Build history of the part. All positions in model axes, mm. A direction names the side the tool comes from. Round coordinates to 2 decimals unless told otherwise and drop trailing zeros. Order: outer loops, then holes, each group sorted by start corner. A loop starts at its lowest first (then second) coordinate and runs counter-clockwise, first axis right, second up. Notation, with made-up numbers: M 32.5,39 L 63.5,39 A33 cw 63.5,69 Z; hole C 25,27.25 d8. An arc over 180 degrees is marked long. One line per item, written item: value. Start each with the question number.
Item 1: Band-saw the part on B-B, the plane z = 0. Give the number of separate pieces and of enclosed holes in the cut face, then the cut area to 3 significant figures.
Item 2: Tool access for faces 4 (the cylindrical face through (3, 30, 0)), 5 (the flat face through (10, 1, 7)): list every direction of +Z, -Z, +X, -X, +Y, -Y with a clear straight run to the whole face (end or side of a thin tool).
Item 3: Band-saw the part on C-C, the plane x = 7. Write the cut outline in (y, z), then the cut area to 3 significant figures.
Item 4: Band-saw the part on D-D, the plane y = 0. Write the cut outline in (x, z).
Item 5: Probe L1, parallel to Y at x = 7.8, z = 0; L2, parallel to Y at x = 2, z = -3.5; L3, parallel to Y at x = 2.4, z = -25. List the from-to ranges inside material, lowest first.
Item 6: Two-plate mould, pull along Y, no slides. Class faces 1 (the flat face through (5, -43, 0)), 2 (the flat face through (5, -1, 31)), 3 (the cylindrical face through (2.71, -4.88, -1.08)): +Y half, -Y half, draft (parallel to the pull), parting line (faces both ways), or undercut.
Item 7: Band-saw the part on A-A, the plane y = 25. Write the cut outline in (x, z), then the cut area to 3 significant figures.
Item 8: Pin check, flat tips, straight feed: pin 1 (5 mm diameter, centred on y = -19, z = 0, fed in from +X); pin 2 (6 mm diameter, centred on y = 0, z = 25, fed in from -X). Stop position of each tip, or through.
```python
from build123d import *

# Parameters (mm, degrees)
SKETCH_1_W                = 62
SKETCH_1_H                = 86
EXTRUDE_1_DEPTH           = 10
CHAMFER_1_SIZE            = 1
HOLE_WIZARD_1_D           = 5.5
HOLE_WIZARD_1_CBORE_D     = 10
HOLE_WIZARD_1_CBORE_DEPTH = 5.5
HOLE_WIZARD_M5_1_D        = 4.2


with BuildPart() as part:
    # 草图1 → 凸台-拉伸1 (new body)
    with BuildSketch(Plane(origin=(0, 0, 0), x_dir=(0, 0, -1), z_dir=(1, 0, 0))):
        Rectangle(SKETCH_1_W, SKETCH_1_H)
    extrude(amount=EXTRUDE_1_DEPTH)

    # 倒角1
    chamfer_1_edges = [part.edges().sort_by_distance(p)[0] for p in [
        (5, 43, 31),
        (5, 43, -31),
        (5, -43, -31),
        (5, -43, 31),
    ]]
    chamfer(chamfer_1_edges, length=CHAMFER_1_SIZE)

    # 打孔尺寸(%根据)内六角圆柱头螺钉的类型1 (through all)
    with Locations(Plane.ZY):
        with Locations((25, 0), (0, -25), (-25, 0), (0, 25), (0, 0)):
            CounterBoreHole(HOLE_WIZARD_1_D / 2, HOLE_WIZARD_1_CBORE_D / 2, HOLE_WIZARD_1_CBORE_DEPTH)

    # M5 螺纹孔1 (through all)
    with Locations(Plane.ZY):
        with Locations((0, 19), (0, -19)):
            Hole(HOLE_WIZARD_M5_1_D / 2)


solid = part.part
```
Output:
1. separate pieces: 6
1. enclosed holes: 0
1. area: 549 mm²
2. face 4: -X
2. face 5: +Z, -Z, +X, +Y, -Y
3. outline: M -43,-30 L -42,-31 L 42,-31 L 43,-30 L 43,30 L 42,31 L -42,31 L -43,30 Z; hole C -25,0 d5.5; hole C -19,0 d4.2; hole C 0,-25 d5.5; hole C 0,0 d5.5; hole C 0,25 d5.5; hole C 19,0 d4.2; hole C 25,0 d5.5
3. area: 5,180 mm²
4. outline: M 0,-31 L 10,-31 L 10,-27.75 L 5.5,-27.75 L 5.5,-30 L 0,-30 Z; M 0,-20 L 5.5,-20 L 5.5,-22.25 L 10,-22.25 L 10,-2.75 L 5.5,-2.75 L 5.5,-5 L 0,-5 Z; M 0,5 L 5.5,5 L 5.5,2.75 L 10,2.75 L 10,22.25 L 5.5,22.25 L 5.5,20 L 0,20 Z; M 0,30 L 5.5,30 L 5.5,27.75 L 10,27.75 L 10,31 L 0,31 Z
5. L1: y = -43 to -27.75, -22.25 to -21.1, -16.9 to -2.75, 2.75 to 16.9, 21.1 to 22.25, 27.75 to 43
5. L2: y = -43 to -28.57, -21.43 to -3.57, 3.57 to 21.43, 28.57 to 43
5. L3: y = -43 to -5, 5 to 43
6. face 1: -Y half
6. face 2: draft
6. face 3: undercut
7. outline: M 0,-31 L 10,-31 L 10,-2.75 L 5.5,-2.75 L 5.5,-5 L 0,-5 Z; M 0,5 L 5.5,5 L 5.5,2.75 L 10,2.75 L 10,31 L 0,31 Z
7. area: 540 mm²
8. pin 1: stops at x = 10
8. pin 2: stops at x = 5.5
